Check sheet for the modelled part. Datum: model origin and axes. Units: mm. Give positions to 0.01 mm unless a question says otherwise; leave off trailing zeros. Write each loop counter-clockwise with the first axis right and the second up, starting at its lowest first coordinate (ties: lowest second). Pieces come first, ordered by that corner, then holes. Notation, with made-up numbers: M 73,82.25 L 115,82.25 A19 ccw 115,101.25 Z; hole C -13.75,-2 d4. An arc over 180 degrees is marked long. Use CSV: the item, a comma, the result in double quotes. Start each with the question number.
1. Cross-section at B-B, the plane x = -135. Enter the section's corners in (y, z).
2. Cross-section at A-A, the plane y = -206.5. Enter the section's corners in (x, z), and give its area (3 significant figures).
3. Scan lines: line 1 (X direction, y = 117, z = -104.5); line 2 (Y direction, x = -25, z = -66); line 3 (Y direction, x = 97.5, z = -163.5). Record each from-to range of solid material in increasing order.
4. Cross-section at C-C, the plane y = -91. Enter the section's corners in (x, z), and give its area (3 significant figures).
5. Depth check by flat-ended pin: P1, Ø13, axis at x = -150, z = -90, coming from the -Y side; P2, Ø9, axis at x = 120, z = -150, coming from the -Y side; P3, Ø4, axis at x = -119.5, z = -35.5, coming from the +Y side. Enter the tip coordinate at first touch or a pass-through.
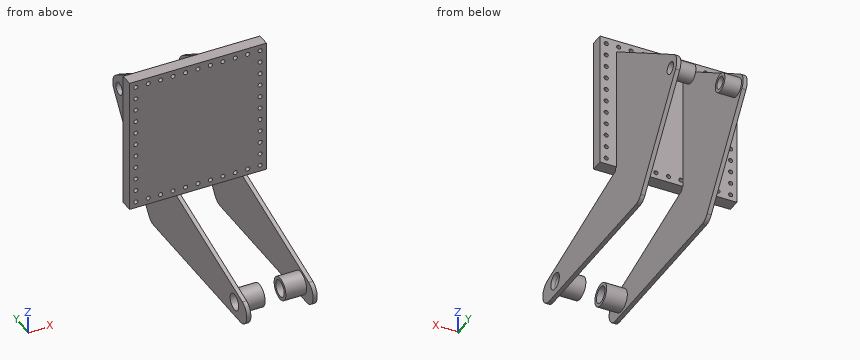
from build123d import *

# Parameters (mm, degrees)
F0_R      = 5
F0_W      = 270
F0_H      = 270
F1_DEPTH  = 30
F4_R      = 20
F4_R_2    = 22.5
F4_R_3    = 15
F5_DEPTH  = 10
F7_R      = 20
F7_R_2    = 22.5
F7_R_3    = 15
F8_DEPTH  = 10
F9_DEPTH  = 40
F10_DEPTH = 40
F13_R     = 27.5
F13_R_2   = 20
F14_DEPTH = 50
F15_R     = 27.5
F15_R_2   = 20
F16_DEPTH = 50


with BuildPart() as f1:
    # F0 (on Front) → F1 (new body)
    with BuildSketch(Plane.XZ):
        Polygon((-165, -165), (-135, -165), (75, -165), (165, -165), (165, 165), (-165, 165), align=None)
        with Locations((-150, -150)):
            Circle(F0_R, mode=Mode.SUBTRACT)
        with Locations((-150, -120)):
            Circle(F0_R, mode=Mode.SUBTRACT)
        with Locations((-120, -150)):
            Circle(F0_R, mode=Mode.SUBTRACT)
        with Locations((-90, -150)):
            Circle(F0_R, mode=Mode.SUBTRACT)
        with Locations((-60, -150)):
            Circle(F0_R, mode=Mode.SUBTRACT)
        with Locations((-30, -150)):
            Circle(F0_R, mode=Mode.SUBTRACT)
        with Locations((0, -150)):
            Circle(F0_R, mode=Mode.SUBTRACT)
        with Locations((30, -150)):
            Circle(F0_R, mode=Mode.SUBTRACT)
        with Locations((60, -150)):
            Circle(F0_R, mode=Mode.SUBTRACT)
        with Locations((90, -150)):
            Circle(F0_R, mode=Mode.SUBTRACT)
        with Locations((120, -150)):
            Circle(F0_R, mode=Mode.SUBTRACT)
        with Locations((150, -150)):
            Circle(F0_R, mode=Mode.SUBTRACT)
        with Locations((150, -120)):
            Circle(F0_R, mode=Mode.SUBTRACT)
        with Locations((-150, -90)):
            Circle(F0_R, mode=Mode.SUBTRACT)
        with Locations((-150, -60)):
            Circle(F0_R, mode=Mode.SUBTRACT)
        with Locations((-150, -30)):
            Circle(F0_R, mode=Mode.SUBTRACT)
        with Locations((-150, 0)):
            Circle(F0_R, mode=Mode.SUBTRACT)
        with Locations((-150, 30)):
            Circle(F0_R, mode=Mode.SUBTRACT)
        with Locations((-150, 60)):
            Circle(F0_R, mode=Mode.SUBTRACT)
        with Locations((-150, 90)):
            Circle(F0_R, mode=Mode.SUBTRACT)
        with Locations((-150, 120)):
            Circle(F0_R, mode=Mode.SUBTRACT)
        with Locations((-150, 150)):
            Circle(F0_R, mode=Mode.SUBTRACT)
        with Locations((-120, 150)):
            Circle(F0_R, mode=Mode.SUBTRACT)
        with Locations((-90, 150)):
            Circle(F0_R, mode=Mode.SUBTRACT)
        with Locations((-60, 150)):
            Circle(F0_R, mode=Mode.SUBTRACT)
        with Locations((-30, 150)):
            Circle(F0_R, mode=Mode.SUBTRACT)
        Rectangle(F0_W, F0_H, mode=Mode.SUBTRACT)
        with Locations((150, -90)):
            Circle(F0_R, mode=Mode.SUBTRACT)
        with Locations((150, -60)):
            Circle(F0_R, mode=Mode.SUBTRACT)
        with Locations((150, -30)):
            Circle(F0_R, mode=Mode.SUBTRACT)
        with Locations((150, 0)):
            Circle(F0_R, mode=Mode.SUBTRACT)
        with Locations((150, 30)):
            Circle(F0_R, mode=Mode.SUBTRACT)
        with Locations((0, 150)):
            Circle(F0_R, mode=Mode.SUBTRACT)
        with Locations((30, 150)):
            Circle(F0_R, mode=Mode.SUBTRACT)
        with Locations((60, 150)):
            Circle(F0_R, mode=Mode.SUBTRACT)
        with Locations((150, 60)):
            Circle(F0_R, mode=Mode.SUBTRACT)
        with Locations((150, 90)):
            Circle(F0_R, mode=Mode.SUBTRACT)
        with Locations((90, 150)):
            Circle(F0_R, mode=Mode.SUBTRACT)
        with Locations((120, 150)):
            Circle(F0_R, mode=Mode.SUBTRACT)
        with BuildLine():
            ThreePointArc((155, 120), (146.4644660941, 116.4644660941), (150, 125))
            ThreePointArc((150, 125), (153.5355339059, 123.5355339059), (155, 120))
        make_face(mode=Mode.SUBTRACT)
        with BuildLine():
            ThreePointArc((155, 150), (153.5355339059, 146.4644660941), (150, 145))
            ThreePointArc((150, 145), (146.4644660941, 153.5355339059), (155, 150))
        make_face(mode=Mode.SUBTRACT)
        Rectangle(F0_W, F0_H)
    extrude(amount=-F1_DEPTH)

    # F4 (on offset) → F5 (join)
    with BuildSketch(Plane.YZ.offset(115)):
        with BuildLine():
            Line((298.8869523608, -37.9796266225), (33.3473250322, 134.1293910905))
            ThreePointArc((33.3473250322, 134.1293910905), (28.2401068156, 134.3266539493), (25.6278477609, 129.9336261577))
            Line((25.6278477609, 129.9336261577), (25.6278477609, -168.7413089787))
            ThreePointArc((25.6278477609, -168.7413089787), (24.6061971658, -171.7699614864), (21.9587533559, -173.5609241394))
            Line((21.9587533559, -173.5609241394), (-296.2802540275, -261.4405704084))
            ThreePointArc((-296.2802540275, -261.4405704084), (-316.0594091243, -294.7644344742), (-286.4742492609, -319.7926826845))
            Line((-286.4742492609, -319.7926826845), (119.3903928782, -319.7926826845))
            ThreePointArc((119.3903928782, -319.7926826845), (133.0674858943, -316.4935651911), (143.7364231218, -307.3218244599))
            Line((143.7364231218, -307.3218244599), (306.9161189768, -80.6833579945))
            ThreePointArc((306.9161189768, -80.6833579945), (312.0534722359, -57.6107428284), (298.8869523608, -37.9796266225))
        make_face()
        with Locations((-258.5189006871, -284.8317994661)):
            Circle(F4_R, mode=Mode.SUBTRACT)
        with Locations((282.5700887333, -63.1542162192)):
            Circle(F4_R_2, mode=Mode.SUBTRACT)
        with Locations((282.5700887333, -63.1542162192)):
            Circle(F4_R_2)
        with Locations((282.5700887333, -63.1542162192)):
            Circle(F4_R_3, mode=Mode.SUBTRACT)
    extrude(amount=F5_DEPTH)

    # F7 (on offset) → F8 (join)
    with BuildSketch(Plane.YZ.offset(-35)):
        with BuildLine():
            ThreePointArc((33.3473250322, 134.1293910905), (28.2401068156, 134.3266539493), (25.6278477609, 129.9336261577))
            Line((25.6278477609, 129.9336261577), (25.6278477609, -168.7413089787))
            ThreePointArc((25.6278477609, -168.7413089787), (24.6061971658, -171.7699614864), (21.9587533559, -173.5609241394))
            Line((21.9587533559, -173.5609241394), (-296.2802540275, -261.4405704084))
            ThreePointArc((-296.2802540275, -261.4405704084), (-316.0594091243, -294.7644344742), (-286.4742492609, -319.7926826845))
            Line((-286.4742492609, -319.7926826845), (119.3903928782, -319.7926826845))
            ThreePointArc((119.3903928782, -319.7926826845), (133.0674858943, -316.4935651911), (143.7364231218, -307.3218244599))
            Line((143.7364231218, -307.3218244599), (306.9161189768, -80.6833579945))
            ThreePointArc((306.9161189768, -80.6833579945), (312.0534722359, -57.6107428284), (298.8869523608, -37.9796266225))
            Line((298.8869523608, -37.9796266225), (33.3473250322, 134.1293910905))
        make_face()
        with Locations((-258.5189006871, -284.8317994661)):
            Circle(F7_R, mode=Mode.SUBTRACT)
        with Locations((282.5700887333, -63.1542162192)):
            Circle(F7_R_2, mode=Mode.SUBTRACT)
        with Locations((282.5700887333, -63.1542162192)):
            Circle(F7_R_2)
        with Locations((282.5700887333, -63.1542162192)):
            Circle(F7_R_3, mode=Mode.SUBTRACT)
    extrude(amount=-F8_DEPTH)

    # F7 (on offset) → F9 (join)
    with BuildSketch(Plane.YZ.offset(-35)):
        with Locations((282.5700887333, -63.1542162192)):
            Circle(F7_R_2)
        with Locations((282.5700887333, -63.1542162192)):
            Circle(F7_R_3, mode=Mode.SUBTRACT)
    extrude(amount=F9_DEPTH)

    # F4 (on offset) → F10 (join)
    with BuildSketch(Plane.YZ.offset(115)):
        with Locations((282.5700887333, -63.1542162192)):
            Circle(F4_R_2)
        with Locations((282.5700887333, -63.1542162192)):
            Circle(F4_R_3, mode=Mode.SUBTRACT)
    extrude(amount=-F10_DEPTH)

    # F13 (on face) → F14 (join)
    with BuildSketch(Plane.YZ.offset(-35)):
        with Locations((-258.5189006871, -284.8317994661)):
            Circle(F13_R)
        with Locations((-258.5189006871, -284.8317994661)):
            Circle(F13_R_2, mode=Mode.SUBTRACT)
    extrude(amount=F14_DEPTH)

    # F15 (on face) → F16 (join)
    with BuildSketch(Plane.YZ.offset(115)):
        with Locations((-258.5189006871, -284.8317994661)):
            Circle(F15_R)
        with Locations((-258.5189006871, -284.8317994661)):
            Circle(F15_R_2, mode=Mode.SUBTRACT)
    extrude(amount=-F16_DEPTH)


solid = f1.part
Worked answers:
1,outline,"M 0,-165 L 30,-165 L 30,165 L 0,165 Z"
2,outline,"M -45,-319.79 L -35,-319.79 L -35,-236.65 L -45,-236.65 Z; M 115,-319.79 L 125,-319.79 L 125,-236.65 L 115,-236.65 Z"
2,area,"1,660 mm^2"
3,line 1,"x = -45 to -35, 115 to 125"
3,line 2,"y = 0 to 30, 260.25 to 267.84, 297.3 to 304.89"
3,line 3,"y = 0 to 30"
4,outline,"M -45,-319.79 L -35,-319.79 L -35,-204.75 L -45,-204.75 Z; M 115,-319.79 L 125,-319.79 L 125,-204.75 L 115,-204.75 Z"
4,area,"2,300 mm^2"
5,P1,"stops at y = 0"
5,P2,"stops at y = 25.63"
5,P3,"stops at y = 30"
